```python
from build123d import *

# Parameters (mm, degrees)
SKETCH003_R  = 1.5
PAD001_DEPTH = 2.4
PAD002_DEPTH = 35.5


with BuildPart() as part:
    # Sketch003 → Pad001 (new body)
    with BuildSketch(Plane.XY):
        with BuildLine():
            ThreePointArc((42.393216, -15.533921), (48.750712, -13.890021), (45, -8.5))
            ThreePointArc((45, 8.5), (36.5, 0), (45, -8.5))
            ThreePointArc((45, 8.5), (48.750712, 13.890021), (42.393216, 15.533921))
            Line((42.393216, 15.533921), (28.910176, 3.949119))
            ThreePointArc((25, 2.5), (27.085031, 2.873932), (28.910176, 3.949119))
            Line((25, 2.5), (-25, 2.5))
            ThreePointArc((-28.910176, 3.949119), (-27.085031, 2.873932), (-25, 2.5))
            Line((-42.393216, 15.533921), (-28.910176, 3.949119))
            ThreePointArc((-42.393216, 15.533921), (-48.750712, 13.890021), (-45, 8.5))
            ThreePointArc((-45, -8.5), (-36.5, 0), (-45, 8.5))
            ThreePointArc((-45, -8.5), (-48.750712, -13.890021), (-42.393216, -15.533921))
            Line((-42.393216, -15.533921), (-28.910176, -3.949119))
            ThreePointArc((-25, -2.5), (-27.085031, -2.873932), (-28.910176, -3.949119))
            Line((-25, -2.5), (25, -2.5))
            ThreePointArc((28.910176, -3.949119), (27.085031, -2.873932), (25, -2.5))
            Line((42.393216, -15.533921), (28.910176, -3.949119))
        make_face()
        with Locations((-45, 12.5)):
            Circle(SKETCH003_R, mode=Mode.SUBTRACT)
        with Locations((-45, -12.5)):
            Circle(SKETCH003_R, mode=Mode.SUBTRACT)
        with Locations((45, 12.5)):
            Circle(SKETCH003_R, mode=Mode.SUBTRACT)
        with Locations((45, -12.5)):
            Circle(SKETCH003_R, mode=Mode.SUBTRACT)
    extrude(amount=PAD001_DEPTH)

    # Sketch004 → Pad002 (join, symmetric)
    with BuildSketch(Plane.YZ):
        with BuildLine():
            ThreePointArc((2.44949, 2.4), (0, 4.4), (-2.44949, 2.4))
            Line((2.44949, 2.4), (-2.44949, 2.4))
        make_face()
    extrude(amount=PAD002_DEPTH, both=True)


solid = part.part
```
Verification items for the finished model (mm, model axes). A direction names the side the tool comes from. Give positions to 0.01 mm unless a question says otherwise; leave off trailing zeros. Order: outer loops, then holes, each group sorted by start corner. A loop starts at its lowest first (then second) coordinate and runs counter-clockwise, first axis right, second up. Notation, with made-up numbers: (64.25, 40.5) - (109.25, 40.5) arc R17 ccw to (109.25, 44.5) - close; hole circle Ø1 at (69.25, 13.25). An arc over 180 degrees is marked (long way). Answer as CSV lines item,"result". Start each with the question number.
Item 1: Gauge pin test, flat ends, axial feed: pin 1 (1 mm diameter, centred on y = -13, z = 3, fed in from +X); pin 2 (2.5 mm diameter, centred on x = 7.5, z = 1, fed in from -Y); pin 3 (1.5 mm diameter, centred on x = -36, z = 2.5, fed in from -Y); pin 4 (2 mm diameter, centred on x = 21.5, z = 4, fed in from -Y) (3 decimals). Record the tip position at first contact, or that the pin passes through.
Item 2: Section check A-A, the plane z = 1.3. Record the boundary of the cut face in (x, y).
Item 3: Section check D-D, the plane y = 12.5. Record the boundary of the cut face in (x, z).
Item 4: Material ranges on L1, parallel to Y at x = -45, z = 0.85; L2, parallel to Y at x = 13, z = 2.1; L3, parallel to Z at x = 39.5, y = 13, recorded low to high.
Item 5: Section check C-C, the plane y = -5. Record the boundary of the cut face in (x, z).
Item 6: Section check B-B, the plane x = 6. Record the boundary of the cut face in (y, z), plus the area to 3 significant figures.
Item 7: Access from +Z, -Z, +X, -X, +Y, -Y to the whole of each face (thin tool, end or side, straight path). Record for faces 1 (the face through (35.746, 9.823, 1.183)), 2 (the face through (0, -2.5, 1)), 3 (the face through (43.5, -12.43, 1.18)).
Item 8: Mould release check, pull along Y, two halves, no side actions. Record for faces 4 (the face through (0, -1, 0)), 5 (the face through (-48.787, -13.788, 1.183)), 6 (the face through (27.057, 2.864, 1.183)): released by +Y, released by -Y, zero draft, split by the parting line, or undercut.
Filled in:
1,pin 1,"through"
1,pin 2,"y = -2.5"
1,pin 3,"y = -10.68"
1,pin 4,"y = -2.245"
2,outline,"(-45, -8.5) arc R4 ccw (long way) to (-42.39, -15.53) - (-28.91, -3.95) arc R6 cw to (-25, -2.5) - (25, -2.5) arc R6 cw to (28.91, -3.95) - (42.39, -15.53) arc R4 ccw (long way) to (45, -8.5) arc R8.5 cw to (45, 8.5) arc R4 ccw (long way) to (42.39, 15.53) - (28.91, 3.95) arc R6 cw to (25, 2.5) - (-25, 2.5) arc R6 cw to (-28.91, 3.95) - (-42.39, 15.53) arc R4 ccw (long way) to (-45, 8.5) arc R8.5 cw to start; hole circle Ø3 at (-45, -12.5); hole circle Ø3 at (-45, 12.5); hole circle Ø3 at (45, -12.5); hole circle Ø3 at (45, 12.5)"
3,outline,"(-49, 0) - (-46.5, 0) - (-46.5, 2.4) - (-49, 2.4) - close; (-43.5, 0) - (-38.86, 0) - (-38.86, 2.4) - (-43.5, 2.4) - close; (38.86, 0) - (43.5, 0) - (43.5, 2.4) - (38.86, 2.4) - close; (46.5, 0) - (49, 0) - (49, 2.4) - (46.5, 2.4) - close"
4,L1,"-16.5 to -14, -11 to -8.5, 8.5 to 11, 14 to 16.5"
4,L2,"-2.5 to 2.5"
4,L3,"0 to 2.4"
5,outline,"(-38.13, 0) - (-30.13, 0) - (-30.13, 2.4) - (-38.13, 2.4) - close; (30.13, 0) - (38.13, 0) - (38.13, 2.4) - (30.13, 2.4) - close"
6,outline,"(-2.5, 0) - (2.5, 0) - (2.5, 2.4) - (2.45, 2.4) arc R2.5 ccw to (-2.45, 2.4) - (-2.5, 2.4) - close"
6,area,"19.3 mm^2"
7,face 1,"+Z, -Z, +Y"
7,face 2,"+Z, -Z, -Y"
7,face 3,"+Z, -Z"
8,face 4,"zero draft"
8,face 5,"undercut"
8,face 6,"released by +Y"
